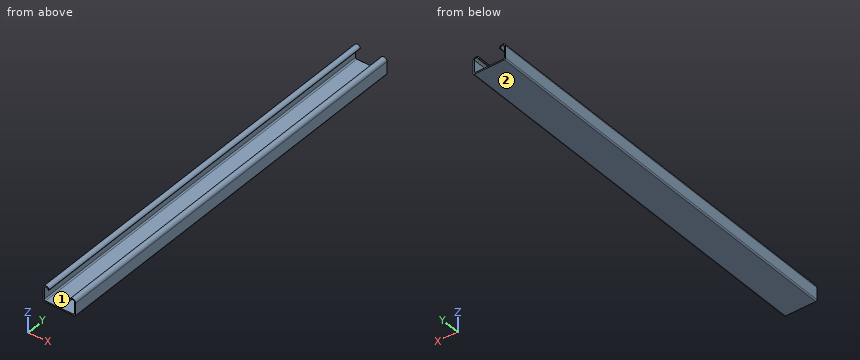
```python
from build123d import *

# Parameters (mm, degrees)
F1_DEPTH    = 250.825
F2_R        = 1.5875
F3_T1_DEPTH = 507.0347591504
F3_T3_DEPTH = 505.1764115156


# Not quite as in the source:
# - a fillet or chamfer that OpenCascade refuses, or shapes differently, is made with other operations: its cross-section is extruded or revolved along the edge and cut away or added


with BuildPart() as f1:
    # F0 (on Front) → F1 (new body, symmetric)
    with BuildSketch(Plane.XZ):
        with BuildLine():
            Line((0, 23.0208111631), (0, 6.3584111631))
            Line((0, 6.3584111631), (41.275, 6.3584111631))
            Line((41.275, 6.3584111631), (41.275, 7.9459111631))
            Line((41.275, 7.9459111631), (41.275, 23.0208111631))
            ThreePointArc((41.275, 23.0208111631), (37.3526007198, 26.9830092528), (33.3510076204, 23.1008085261))
            Line((33.3510076204, 23.1008085261), (34.7028554043, 23.1008085261))
            ThreePointArc((34.7028554043, 23.1008085261), (36.7966084578, 25.5802875082), (39.6875, 24.1057150403))
            Line((39.6875, 24.1057150403), (39.6875, 23.1008085261))
            Line((39.6875, 23.1008085261), (39.6875, 7.9459111631))
            Line((39.6875, 7.9459111631), (1.5875, 7.9459111631))
            Line((1.5875, 7.9459111631), (1.5875, 24.1057150403))
            ThreePointArc((1.5875, 24.1057150403), (4.4783915422, 25.5802875082), (6.5721445957, 23.1008085261))
            Line((6.5721445957, 23.1008085261), (7.9239923796, 23.1008085261))
            ThreePointArc((7.9239923796, 23.1008085261), (3.9223992802, 26.9830092528), (0, 23.0208111631))
        make_face()
    extrude(amount=F1_DEPTH, both=True)

    # F2
    f2_edges = [f1.edges().sort_by_distance(p)[0] for p in [
        (39.6875, 0, 7.945911),
        (1.5875, 0, 7.945911),
        (0, 0, 6.358411),
        (41.275, 0, 6.358411),
    ]]
    fillet(f2_edges, radius=F2_R)

    # F3: fillet of radius 0.8255 on 4 edges, made by hand

    # F3_s2 → F3_t1 (cut)
    with BuildSketch(Plane.XZ.offset(-253.5173795752)):
        with BuildLine():
            ThreePointArc((33.5188726746, 24.1645973059), (33.6466023062, 23.4339961952), (34.309232534, 23.1008085261))
            Line((34.309232534, 23.1008085261), (33.3510076204, 23.1008085261))
            ThreePointArc((33.3510076204, 23.1008085261), (33.3986304583, 23.6384325571), (33.5188726746, 24.1645973059))
        make_face()
        with BuildLine():
            ThreePointArc((7.7561273254, 24.1645973059), (7.6283976938, 23.4339961952), (6.965767466, 23.1008085261))
            Line((6.965767466, 23.1008085261), (7.9239923796, 23.1008085261))
            ThreePointArc((7.9239923796, 23.1008085261), (7.8763695417, 23.6384325571), (7.7561273254, 24.1645973059))
        make_face()
    extrude(amount=F3_T1_DEPTH, mode=Mode.SUBTRACT)

    # F3_s4 → F3_t3 (cut)
    with BuildSketch(Plane.XZ.offset(-252.5882057578)):
        with BuildLine():
            ThreePointArc((33.9975731012, 23.1008085261), (34.4985175119, 23.2701797679), (34.7939002584, 23.7087922999))
            ThreePointArc((34.7939002584, 23.7087922999), (34.7304213855, 23.4074893696), (34.7028554043, 23.1008085261))
            Line((34.7028554043, 23.1008085261), (33.9975731012, 23.1008085261))
        make_face()
        with BuildLine():
            ThreePointArc((7.2774268988, 23.1008085261), (6.7764824881, 23.2701797679), (6.4810997416, 23.7087922999))
            ThreePointArc((6.4810997416, 23.7087922999), (6.5445786145, 23.4074893696), (6.5721445957, 23.1008085261))
            Line((6.5721445957, 23.1008085261), (7.2774268988, 23.1008085261))
        make_face()
    extrude(amount=F3_T3_DEPTH, mode=Mode.SUBTRACT)


solid = f1.part
```
Can you work these out from the model? Positions are in its coordinate system, mm. Face numbers are marked on the shaded views. Round coordinates to 2 decimals unless told otherwise and drop trailing zeros. Loops run counter-clockwise (first coordinate to the right, second up) from the corner with the lowest first, then second, coordinate; pieces in that order, holes last. Notation, with made-up numbers: (39, 27.25) -> (52, 27.25) arc R21 ccw to (52, 39.25) -> close; hole circle Ø9 at (30.5, -38). An arc over 180 degrees is marked (long way). One line per item, written item: value. Start each with the question number.
1. If we section it at A-A, the plane z = 15.75: Write out the boundary of the cut face in (x, y) (1 decimal), then the cut area to 3 significant figures.
2. If I drill on probe 1 along Z at (x, y) = (7, -82.5); probe 2 along X at (y, z) = (131, 16.25) (1 decimal); probe 3 along X at (y, z) = (-120, 25.25), over which ranges is the centre line in solid material (lowest first)?
3. For pin 1 (6 mm diameter, centred on x = 32, y = 130, fed in from +Z), with a flat end and sliding along its axis, tell me the tip position at first contact or that it passes through.
4. If we section it at B-B, the plane y = -167: Write out the boundary of the cut face in (x, z) (1 decimal).
5. If we mould it in two halves opening along X, with no side actions, what happens to the marked faces 1 and 2? For each: pulls with the +X half, pulls with the -X half, needs draft (parallel to the pull), parting line crosses it, or undercut.
6. If we section it at C-C, the plane x = 23: Write out the boundary of the cut face in (y, z) (3 decimals).
Calculated:
1. outline: (0, -250.8) -> (1.6, -250.8) -> (1.6, 250.8) -> (0, 250.8) -> close; (39.7, -250.8) -> (41.3, -250.8) -> (41.3, 250.8) -> (39.7, 250.8) -> close
1. area: 1,590 mm²
2. probe 1: z = 6.36 to 7.95, 23.15 to 25.57
2. probe 2: x = 0 to 1.6, 39.7 to 41.3
2. probe 3: x = 0.69 to 2.6, 5.32 to 7.24, 34.04 to 35.95, 38.67 to 40.59
3. pin 1: stops at z = 26.24
4. outline: (0, 7.9) arc R1.6 ccw to (1.6, 6.4) -> (39.7, 6.4) arc R1.6 ccw to (41.3, 7.9) -> (41.3, 23) arc R4 ccw to (33.5, 24.2) arc R0.8 ccw to (34.2, 23.1) arc R0.8 ccw to (34.8, 23.7) arc R2.6 cw to (39.7, 24.1) -> (39.7, 9.5) arc R1.6 cw to (38.1, 7.9) -> (3.2, 7.9) arc R1.6 cw to (1.6, 9.5) -> (1.6, 24.1) arc R2.6 cw to (6.5, 23.7) arc R0.8 ccw to (7.1, 23.1) arc R0.8 ccw to (7.8, 24.2) arc R4 ccw to (0, 23) -> close
5. face 1: undercut
5. face 2: needs draft
6. outline: (-250.825, 6.358) -> (250.825, 6.358) -> (250.825, 7.946) -> (-250.825, 7.946) -> close
